Geometry: final body of the model. Coordinates: model frame, mm. A direction names the side the tool comes from. Round coordinates to 2 decimals unless told otherwise and drop trailing zeros. Loops run counter-clockwise (first coordinate to the right, second up) from the corner with the lowest first, then second, coordinate; pieces in that order, holes last. Notation, with made-up numbers: (44.5, -9) - (76.5, -9) arc R22 ccw to (76.5, -3) - close; hole circle Ø6 at (-39.5, 4). An arc over 180 degrees is marked (long way). Use CSV: the item, a comma, the result in double quotes.
Autodesk Inventor part; units mm, degrees
ref_plane "YZ Plane" through (0, 0, 0) normal (1, 0, 0) x (0, 1, 0)
ref_plane "XZ Plane" through (0, 0, 0) normal (0, 1, 0) x (-1, 0, 0)
ref_plane "XY Plane" through (0, 0, 0) normal (0, 0, 1) x (1, 0, 0)
sketch "Sketch1" plane through (0, 0, 0) normal (0, 0, 1) x (1, 0, 0)
  line L0 (44.5, 57.5) -> (-44.5, 57.5)
  line L1 (-44.5, 57.5) -> (-44.5, -57.5)
  line L2 (-44.5, -57.5) -> (44.5, -57.5)
  line L3 (44.5, -57.5) -> (44.5, 57.5)
  point P0 (0, 0)
  dimension "d0" = 89
  dimension "d3" = 115
  dimension "d4" = 57.5
  dimension "d5" = 44.5
extrude "Extrusion1" add sketch "Sketch1" along normal blind 5
sketch "Sketch2" plane through (0, 0, 5) normal (0, 0, 1) x (1, 0, 0)
  line L0 (-44.5, -52.5) -> (44.5, -52.5)
  line L1 (44.5, -52.5) -> (44.5, -57.5)
  line L2 (44.5, -57.5) -> (-44.5, -57.5)
  line L3 (-44.5, -57.5) -> (-44.5, -52.5)
  point P0 (0, 0)
  dimension "d8" = 89
  dimension "d9" = 5
extrude "Extrusion2" add sketch "Sketch2" along normal blind 39
properties part number "back_plate"
Item 1: Section B-B on z = 15.5. Return the cut outline in (x, y), plus the area to 3 significant figures.
Final values:
outline,"(-44.5, -57.5) - (44.5, -57.5) - (44.5, -52.5) - (-44.5, -52.5) - close"
area,"445 mm²"
Item 2: Section A-A on x = 25.5. Return the cut outline in (y, z).
Final values:
outline,"(-57.5, 0) - (57.5, 0) - (57.5, 5) - (-52.5, 5) - (-52.5, 44) - (-57.5, 44) - close"
Item 3: Material intervals for line 1 (Y direction, x = 38, z = 6.5); line 2 (Z direction, x = -39, y = 50), sorted ascending.
Final values:
line 1,"y = -57.5 to -52.5"
line 2,"z = 0 to 5"
Item 4: Reachability of faces 1 (the flat face through (-44.5, -8, 4)), 2 (the flat face through (-1, -52.5, 24)) from +Z, -Z, +X, -X, +Y, -Y: full face, straight path, thin tool, end or side. Return the list, or none.
Final values:
face 1,"+Z, -Z, -X, +Y, -Y"
face 2,"+Z, +X, -X, +Y"
Item 5: Section C-C on y = 20. Return the cut outline in (x, z), plus the area to 3 significant figures.
Final values:
outline,"(-44.5, 0) - (44.5, 0) - (44.5, 5) - (-44.5, 5) - close"
area,"445 mm²"
Item 6: Pin query (flat end, axial travel): P1, Ø1, axis at x = 21.5, y = 15.5, coming from the +Z side; P2, Ø8, axis at x = 19, y = 8, coming from the -Z side; P3, Ø6, axis at x = -15, z = 17, coming from the +Y side. Return the tip coordinate at first contact, or that it passes through.
Final values:
P1,"stops at z = 5"
P2,"stops at z = 0"
P3,"stops at y = -52.5"
